Job drawing, mm, ordinate dimensions from the low corner. One solid piece. Coordinates: 2 decimals unless noted, no trailing zeros. Order: outer loops, then holes, each group sorted by start corner. A loop starts at its lowest first (then second) coordinate and runs counter-clockwise, first axis right, second up. Notation, with made-up numbers: M 80.5,86 L 134.5,86 A14 ccw 134.5,111 Z; hole C 43.5,-36 d5. An arc over 180 degrees is marked long. Write item = value, one per line. Start each with the question number.
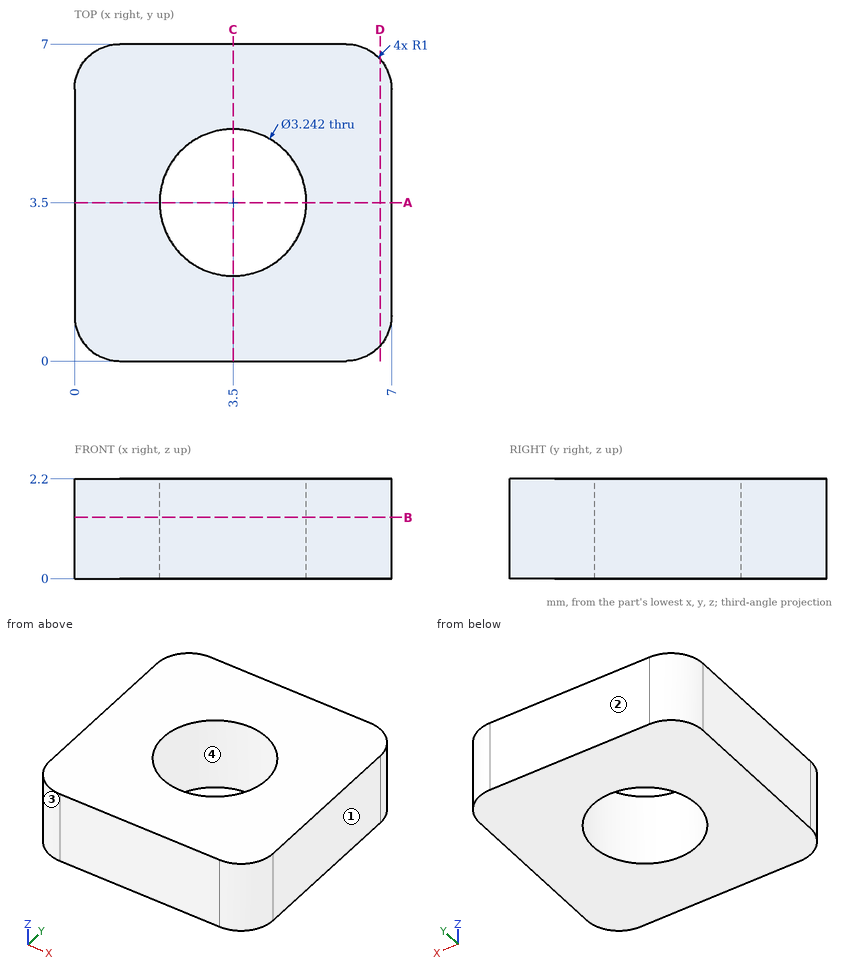
Item 1: Cut at A-A, the plane y = 3.5. Write the cut outline in (x, z), and give its area (3 significant figures).
Item 2: Pull direction Y, two halves, no side cores. Call the marked faces 1, 2, 3 and 4: pulls with the +Y half, pulls with the -Y half, needs draft (parallel to the pull), parting line crosses it, or undercut.
Item 3: Wall check: line 1 along Y through (x, z) = (3.5, 1.15); line 2 along X through (y, z) = (2.25, 2.15). Give the ranges that are in metal, low to high. Write a range as [from, to].
Item 4: Cut at D-D, the plane x = 6.75. Write the cut outline in (y, z).
Item 5: Cut at B-B, the plane z = 1.35. Write the cut outline in (x, y).
Item 6: Flat gauge pin, fed straight in: pin 1 (2.5 mm diameter, centred on x = 3.5, y = 3.5, fed in from -Z). Where does the tip first touch, or does it go through?
Filled sheet:
q1.outline = M 0,0 L 1.88,0 L 1.88,2.2 L 0,2.2 Z; M 5.12,0 L 7,0 L 7,2.2 L 5.12,2.2 Z
q1.area = 8.27 mm2
q2.face_1 = needs draft
q2.face_2 = pulls with the +Y half
q2.face_3 = pulls with the -Y half
q2.face_4 = undercut
q3.line_1 = [0, 1.88], [5.12, 7]
q3.line_2 = [0, 2.47], [4.53, 7]
q4.outline = M 0.34,0 L 6.66,0 L 6.66,2.2 L 0.34,2.2 Z
q5.outline = M 0,1 A1 ccw 1,0 L 6,0 A1 ccw 7,1 L 7,6 A1 ccw 6,7 L 1,7 A1 ccw 0,6 Z; hole C 3.5,3.5 d3.24
q6.pin_1 = through
